Part model, mm, in its own coordinate system. Round coordinates to 2 decimals unless told otherwise and drop trailing zeros. Loops run counter-clockwise (first coordinate to the right, second up) from the corner with the lowest first, then second, coordinate; pieces in that order, holes last. Notation, with made-up numbers: (77, 38.5) -> (119, 38.5) arc R12 ccw to (119, 49.5) -> close; hole circle Ø5 at (-34.5, 42.25). An arc over 180 degrees is marked (long way). Use a Markdown table: item, result. Add a question column.
Item 1: Cut at D-D, the plane y = -10.5. List the corners of the cut face in (x, z).
Item 2: Flat gauge pins, fed straight in: pin 1 (3 mm diameter, centred on y = 6, z = 4, fed in from +X); pin 2 (1 mm diameter, centred on y = -1.5, z = 4, fed in from +X); pin 3 (1.5 mm diameter, centred on x = -4, z = 3, fed in from +Y). Where does each tip first touch, or does it go through?
Item 3: Probe line 1 (X direction, y = 7, z = 2.5); line 2 (Y direction, x = -7.5, z = 2.45). List the from-to ranges inside material, lowest first. Write a range as [from, to].
Item 4: Cut at A-A, the plane z = 3.3. List the corners of the cut face in (x, y), plus the area to 3 significant figures.
Item 5: Cut at C-C, the plane x = -10. List the corners of the cut face in (y, z), plus the area to 3 significant figures.
Item 6: Cut at B-B, the plane y = 6.5. List the corners of the cut face in (x, z).
```python
from build123d import *

# Parameters (mm, degrees)
F0_R     = 16
F1_DEPTH = 5


with BuildPart() as f1:
    # F0 (on Top) → F1 (new body)
    with BuildSketch(Plane.XY):
        Circle(F0_R)
        with BuildLine():
            Line((5.95, -7.5), (-5.95, -7.5))
            ThreePointArc((-5.95, -7.5), (-8.5960155108, -8.5960155108), (-7.5, -5.95))
            Line((-7.5, -5.95), (-7.5, 5.95))
            ThreePointArc((-7.5, 5.95), (-8.5960155108, 8.5960155108), (-5.95, 7.5))
            Line((-5.95, 7.5), (5.95, 7.5))
            ThreePointArc((5.95, 7.5), (7.5, 9.05), (9.05, 7.5))
            ThreePointArc((9.05, 7.5), (8.5960155108, 6.4039844892), (7.5, 5.95))
            Line((7.5, 5.95), (7.5, -5.95))
            ThreePointArc((7.5, -5.95), (8.5960155108, -6.4039844892), (9.05, -7.5))
            ThreePointArc((9.05, -7.5), (7.5, -9.05), (5.95, -7.5))
        make_face(mode=Mode.SUBTRACT)
        with BuildLine():
            ThreePointArc((-7.5, -5.95), (-6.4039844892, -6.4039844892), (-5.95, -7.5))
            Line((-5.95, -7.5), (5.95, -7.5))
            ThreePointArc((5.95, -7.5), (6.4039844892, -6.4039844892), (7.5, -5.95))
            Line((7.5, -5.95), (7.5, 5.95))
            ThreePointArc((7.5, 5.95), (6.4039844892, 6.4039844892), (5.95, 7.5))
            Line((5.95, 7.5), (-5.95, 7.5))
            ThreePointArc((-5.95, 7.5), (-6.4039844892, 6.4039844892), (-7.5, 5.95))
            Line((-7.5, 5.95), (-7.5, -5.95))
        make_face()
    extrude(amount=F1_DEPTH)


solid = f1.part
```
A:
| question | item | result |
|---|---|---|
| 1 | outline | (-12.07, 0) -> (12.07, 0) -> (12.07, 5) -> (-12.07, 5) -> close |
| 2 | pin 1 | stops at x = 15.35 |
| 2 | pin 2 | stops at x = 15.97 |
| 2 | pin 3 | stops at y = 15.67 |
| 3 | line 1 | x = [-14.39, -8.97], [-6.03, 6.03], [8.97, 14.39] |
| 3 | line 2 | y = [-14.13, -9.05], [-5.95, 5.95], [9.05, 14.13] |
| 4 | outline | circle Ø32 at (0, 0); hole circle Ø3.1 at (-7.5, -7.5); hole circle Ø3.1 at (-7.5, 7.5); hole circle Ø3.1 at (7.5, -7.5); hole circle Ø3.1 at (7.5, 7.5) |
| 4 | area | 774 mm^2 |
| 5 | outline | (-12.49, 0) -> (12.49, 0) -> (12.49, 5) -> (-12.49, 5) -> close |
| 5 | area | 125 mm^2 |
| 6 | outline | (-14.62, 0) -> (-8.68, 0) -> (-8.68, 5) -> (-14.62, 5) -> close; (-6.32, 0) -> (6.32, 0) -> (6.32, 5) -> (-6.32, 5) -> close; (8.68, 0) -> (14.62, 0) -> (14.62, 5) -> (8.68, 5) -> close |
